The model under review builds one solid part; all positions refer to its coordinate system, in mm. Round coordinates to 2 decimals unless told otherwise and drop trailing zeros. Write each loop counter-clockwise with the first axis right and the second up, starting at its lowest first coordinate (ties: lowest second). Pieces come first, ordered by that corner, then holes. Notation, with made-up numbers: (-27.5, -17.5) - (-12.5, -17.5) arc R9 ccw to (-12.5, -7.5) - close; hole circle Ø8 at (63.25, -9). An arc over 180 degrees is marked (long way). One line per question, with ' | ' between items. Start each with the question number.
```python
from build123d import *

# Parameters (mm, degrees)
BOSS_EXTRUDE1_DEPTH = 164.30625
CUT_EXTRUDE1_DEPTH  = 205.500810654
CUT_EXTRUDE2_DEPTH  = 205.500810654


with BuildPart() as part:
    # Sketch3 → Boss-Extrude1 (new body)
    with BuildSketch(Plane(origin=(0, 0, 0), x_dir=(1, 0, 0), z_dir=(0, 1, 0))):
        with BuildLine():
            Line((-54.4068, 0), (-54.2036, 50.8))
            Line((-54.2036, 50.8), (54.2036, 50.8))
            Line((54.2036, 50.8), (54.4068, 0))
            ThreePointArc((54.4068, 0), (0, -54.4068), (-54.4068, 0))
        make_face()
    extrude(amount=BOSS_EXTRUDE1_DEPTH)

    # Sketch6 → Cut-Extrude1 (cut, through all)
    with BuildSketch(Plane(origin=(-54.405929505, 0, -0.217623718), x_dir=(-0.003999968000384008, 0, 0.9999920000959988), z_dir=(-0.9999920000959988, 0, -0.003999968000384008))):
        Polygon((-50.582780939, 119.0752), (0.217625459, 164.30625), (-50.582780939, 164.30625), align=None)
    extrude(amount=-CUT_EXTRUDE1_DEPTH, mode=Mode.SUBTRACT)

    # Sketch6_3 → Cut-Extrude2 (cut, through all)
    with BuildSketch(Plane(origin=(-54.405929505, 0, -0.217623718), x_dir=(-0.003999968000384008, 0, 0.9999920000959988), z_dir=(-0.9999920000959988, 0, -0.003999968000384008))):
        Polygon((-50.582780939, 119.0752), (0.217625459, 164.30625), (-50.582780939, 164.30625), align=None)
        Polygon((-50.582780939, 164.30625), (0.217625459, 164.30625), (0.217625459, 170.743194309), (-79.741095166, 170.743194309), (-79.741095166, 119.0752), (-50.582780939, 119.0752), align=None)
    extrude(amount=-CUT_EXTRUDE2_DEPTH, mode=Mode.SUBTRACT)


solid = part.part
```
1. Add section B-B, the plane y = 108.5. Write out the cut boundary in (x, z).
2. Clearance check with flat-ended pins moving along their axes: P1, Ø6, axis at y = 126.5, z = -26.5, coming from the +X side; P2, Ø6, axis at x = 31, y = 84, coming from the +Z side; P3, Ø5, axis at x = -16, y = 94.5, coming from the +Z side. State where each tip first meets the part, or that it passes through.
3. Wall thickness on line 1 along X through (y, z) = (65, -8); line 2 along X through (y, z) = (120, -39.5); line 3 along Z through (x, y) = (-5, 92): over which ranges is each line inside the solid? List them lowest first. Write a range as [from, to].
4. Add section D-D, the plane x = 35. Write out the cut boundary in (y, z), then the cut area to 3 significant figures.
5. The part is to be moulded in two halves that separate along Z. For faces 1 (the face through (1, 164.306, 21)), 2 (the face through (1.196, 81.003, 54.394)), 3 (the face through (-1, 59, -50.8)), say which applies: pulls with the +Z half, pulls with the -Z half, needs draft (parallel to the pull), parting line crosses it, or undercut.
6. Add section C-C, the plane z = -9. Write out the cut boundary in (x, y), then the cut area to 3 significant figures.
7. Add section A-A, the plane x = 0. Write out the cut boundary in (y, z).
Geometry check:
1) outline: (-54.41, 0) - (-54.2, -50.8) - (54.2, -50.8) - (54.41, 0) arc R54.41 ccw to start
2) P1: stops at x = 54.31 | P2: stops at z = 46.65 | P3: stops at z = 52.71
3) line 1: x = [-54.37, 54.37] | line 2: x = [-54.25, 54.25] | line 3: z = [-50.8, 54.18]
4) outline: (0, -50.8) - (119.08, -50.8) - (119.08, -50.44) - (164.31, 0.36) - (164.31, 41.65) - (0, 41.65) - close | area: 14,000 mm2
5) face 1: needs draft | face 2: pulls with the +Z half | face 3: pulls with the -Z half
6) outline: (-54.37, 0) - (54.37, 0) - (54.37, 155.91) - (-54.37, 156.29) - close | area: 17,000 mm2
7) outline: (0, -50.8) - (119.08, -50.8) - (119.08, -50.58) - (164.31, 0.22) - (164.31, 54.41) - (0, 54.41) - close
